Part model, mm, in its own coordinate system. Face numbers are marked on the shaded views. Round coordinates to 2 decimals unless told otherwise and drop trailing zeros. Write each loop counter-clockwise with the first axis right and the second up, starting at its lowest first coordinate (ties: lowest second). Pieces come first, ordered by that corner, then holes. Notation, with made-up numbers: (37.5, 18.5) -> (47.5, 18.5) arc R25 cw to (47.5, 51.5) -> close; hole circle Ø4 at (63, 87). An arc over 180 degrees is marked (long way). Use CSV: the item, a comma, the result in double quotes. Start each with the question number.
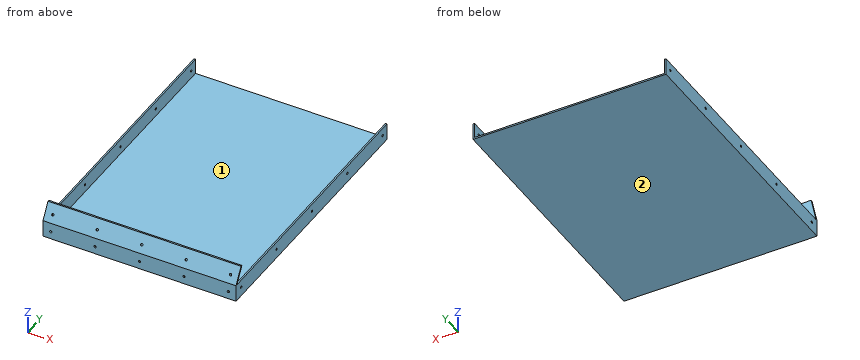
```python
from build123d import *

# Parameters (mm, degrees)
SKETCH063_W     = 251
SKETCH063_H     = 42
PAD011_DEPTH    = 350
POCKET027_DEPTH = 251.001
POCKET028_DEPTH = 251.001
SKETCH039_W     = 2
SKETCH039_H     = 348
PAD034_DEPTH    = 20
SKETCH091_R     = 1.5
POCKET049_DEPTH = 5
SKETCH092_R     = 1.5
POCKET050_DEPTH = 5
SKETCH093_R     = 1.5
POCKET051_DEPTH = 251.001


with BuildPart() as part:
    # Sketch063 (on Face1 of Binder032) → Pad011 (new body)
    with BuildSketch(Plane(origin=(0, -0.1, 0), x_dir=(-1, 0, 0), z_dir=(0, 1, 0))):
        with Locations((-752.5, -204.170471)):
            Rectangle(SKETCH063_W, SKETCH063_H)
    extrude(amount=PAD011_DEPTH)

    # Sketch064 (on Face1 of Pad011) → Pocket027 (cut, through all)
    with BuildSketch(Plane.YZ.offset(878)):
        Polygon((-0.1, -183.170471), (11.464042, -183.170471), (-0.1, -203.2), align=None)
    extrude(amount=-POCKET027_DEPTH, mode=Mode.SUBTRACT)

    # Sketch038 (on Face1 of Pocket027) → Pocket028 (cut, through all)
    with BuildSketch(Plane.YZ.offset(878)):
        Polygon((13.464042, -183.170471), (1.9, -203.2), (1.9, -223.170471), (349.9, -223.170471), (349.9, -183.170471), align=None)
    extrude(amount=-POCKET028_DEPTH, mode=Mode.SUBTRACT)

    # Sketch039 (on Face5 of Pocket028) → Pad034 (join)
    with BuildSketch(Plane.XY.offset(-223.170471)):
        with Locations((877, 175.9)):
            Rectangle(SKETCH039_W, SKETCH039_H)
        with Locations((628, 175.9)):
            Rectangle(SKETCH039_W, SKETCH039_H)
    extrude(amount=PAD034_DEPTH)

    # Sketch091 (on Face5 of Pad034) → Pocket049 (cut)
    with BuildSketch(Plane(origin=(0, 87.913136, -50.75662), x_dir=(1, 0, 0), z_dir=(0, -0.866026, 0.5))):
        with Locations((868, -166.026408)):
            Circle(SKETCH091_R)
        with Locations((810.25, -166.026408)):
            Circle(SKETCH091_R)
        with Locations((752.5, -166.026408)):
            Circle(SKETCH091_R)
        with Locations((694.75, -166.026408)):
            Circle(SKETCH091_R)
        with Locations((637, -166.026408)):
            Circle(SKETCH091_R)
    extrude(amount=-POCKET049_DEPTH, mode=Mode.SUBTRACT)

    # Sketch092 (on Face18 of Pocket049) → Pocket050 (cut)
    with BuildSketch(Plane.XZ.offset(0.1)):
        with Locations((868, -215.170471)):
            Circle(SKETCH092_R)
        with Locations((810.25, -215.170471)):
            Circle(SKETCH092_R)
        with Locations((752.5, -215.170471)):
            Circle(SKETCH092_R)
        with Locations((694.75, -215.170471)):
            Circle(SKETCH092_R)
        with Locations((637, -215.170471)):
            Circle(SKETCH092_R)
    extrude(amount=-POCKET050_DEPTH, mode=Mode.SUBTRACT)

    # Sketch093 (on Face10 of Pocket050) → Pocket051 (cut, through all)
    with BuildSketch(Plane(origin=(627, 0, 0), x_dir=(0, -1, 0), z_dir=(-1, 0, 0))):
        with Locations((-11.917049, -213.170471)):
            Circle(SKETCH093_R)
        with Locations((-93.912786, -213.170471)):
            Circle(SKETCH093_R)
        with Locations((-175.908524, -213.170471)):
            Circle(SKETCH093_R)
        with Locations((-257.904262, -213.170471)):
            Circle(SKETCH093_R)
        with Locations((-339.9, -213.170471)):
            Circle(SKETCH093_R)
    extrude(amount=-POCKET051_DEPTH, mode=Mode.SUBTRACT)


solid = part.part
```
1. Band-saw the part on B-B (y = 56). List the corners of the cut face in (x, z), then the cut area to 3 significant figures.
2. Flat gauge pins, fed straight in: pin 1 (2 mm diameter, centred on x = 784.5, z = -219.5, fed in from +Y); pin 2 (22 mm diameter, centred on x = 780.5, z = -212, fed in from +Y); pin 3 (1 mm diameter, centred on x = 877, y = 91.5, fed in from +Z); pin 4 (2.5 mm diameter, centred on y = 257.9, z = -213.17, fed in from +X). Where does each tip first touch, or does it go through?
3. Drill centre lines: line 1 along X through (y, z) = (267.5, -207); line 2 along Z through (x, y) = (810, 262); line 3 along Z through (x, y) = (637, 0). Where is each one in solid material? Low to high. Write a range as [from, to].
4. Band-saw the part on A-A (x = 657). List the corners of the cut face in (y, z), then the cut area to 3 significant figures.
5. Pull direction X, two halves, no side cores. Call the marked faces 1 and 2: released by +X, released by -X, zero draft, split by the parting line, or undercut.
Answers below:
1,outline,"(627, -225.17) -> (878, -225.17) -> (878, -203.17) -> (876, -203.17) -> (876, -223.17) -> (629, -223.17) -> (629, -203.17) -> (627, -203.17) -> close"
1,area,"582 mm^2"
2,pin 1,"stops at y = 1.9"
2,pin 2,"stops at y = 3.17"
2,pin 3,"stops at z = -203.17"
2,pin 4,"passes through"
3,line 1,"x = [627, 629], [876, 878]"
3,line 2,"z = [-225.17, -223.17]"
3,line 3,"z = [-225.17, -216.67], [-213.67, -203.03]"
4,outline,"(-0.1, -225.17) -> (349.9, -225.17) -> (349.9, -223.17) -> (1.9, -223.17) -> (1.9, -203.2) -> (13.46, -183.17) -> (11.46, -183.17) -> (-0.1, -203.2) -> close"
4,area,"780 mm^2"
5,face 1,"undercut"
5,face 2,"zero draft"
